For this review, take the finished solid that the model builds, in its own axes (mm). Coordinates: 2 decimals unless noted, no trailing zeros. Write each loop counter-clockwise with the first axis right and the second up, starting at its lowest first coordinate (ties: lowest second). Pieces come first, ordered by that corner, then holes.
1) We need section A-A on y = 0. Write out the cut boundary in (x, z).
2) Insertion check: P1, Ø1, axis at x = 78.5, y = -3, coming from the -Z side; P2, Ø0.8, axis at x = 37.5, z = 7, coming from the -Y side; P3, Ø6, axis at x = 48, y = 4.5, coming from the +Z side. Each pin has a flat end and moves straight along its axis. Give the tip position at first contact, or say it passes through.
3) We need section D-D on x = 24.5. Write out the cut boundary in (y, z), then the cut area to 3 significant figures.
4) We need section B-B on x = 119. Write out the cut boundary in (y, z).
5) We need section C-C on z = 2. Write out the cut boundary in (x, y), then the cut area to 3 significant figures.
6) To check wall thickness, follow line 1 along Z through (x, y) = (64, 0.25); line 2 along Y through (x, z) = (28, 7.25); line 3 along Y through (x, z) = (20.5, -5). State the ranges of each line that lie inside material, in increasing order.
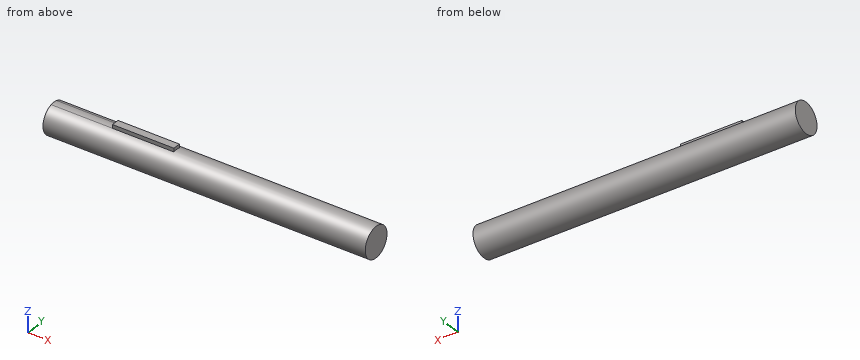
from build123d import *

# Parameters (mm, degrees)
F0_W     = 133.35
F0_H     = 6.35
F3_DEPTH = 50.8
F5_DEPTH = 25.4


with BuildPart() as f1:
    # F0 (on Front) → F1 (revolve)
    with BuildSketch(Plane.XZ):
        with Locations((62.719703, 3.175)):
            Rectangle(F0_W, F0_H)
    revolve(axis=Axis((62.719703, 0, 0), (1, 0, 0)))

    # F2 (on face) → F3 (join)
    with BuildSketch(Plane(origin=(-3.955297, 0, 0), x_dir=(0, -1, 0), z_dir=(-1, 0, 0))):
        with BuildLine():
            Line((-1.5875, 7.672361), (-1.5875, 6.148361))
            ThreePointArc((-1.5875, 6.148361), (0, 6.35), (1.5875, 6.148361))
            Line((1.5875, 6.148361), (1.5875, 7.672361))
            Line((1.5875, 7.672361), (-1.5875, 7.672361))
        make_face()
    extrude(amount=-F3_DEPTH)

    # F4 (on face) → F5 (cut)
    with BuildSketch(Plane(origin=(-3.955297, 0, 0), x_dir=(0, -1, 0), z_dir=(-1, 0, 0))):
        with BuildLine():
            ThreePointArc((-1.5875, 6.148361), (0, 6.35), (1.5875, 6.148361))
            Line((1.5875, 6.148361), (1.5875, 7.672361))
            Line((1.5875, 7.672361), (-1.5875, 7.672361))
            Line((-1.5875, 7.672361), (-1.5875, 6.148361))
        make_face()
    extrude(amount=-F5_DEPTH, mode=Mode.SUBTRACT)


solid = f1.part
Result:
1. outline: (-3.96, -6.35) - (129.39, -6.35) - (129.39, 6.35) - (46.84, 6.35) - (46.84, 7.67) - (21.44, 7.67) - (21.44, 6.35) - (-3.96, 6.35) - close
2. P1: stops at z = -5.84
2. P2: stops at y = -1.59
2. P3: stops at z = 6.17
3. outline: (-1.59, 6.15) arc R6.35 ccw (long way) to (1.59, 6.15) - (1.59, 7.67) - (-1.59, 7.67) - close
3. area: 131 mm2
4. outline: circle Ø12.7 at (0, 0)
5. outline: (-3.96, -6.03) - (129.39, -6.03) - (129.39, 6.03) - (-3.96, 6.03) - close
5. area: 1,610 mm2
6. line 1: z = -6.35 to 6.35
6. line 2: y = -1.59 to 1.59
6. line 3: y = -3.91 to 3.91
